Input: part model. Units: mm. Frame: model coordinates. A direction names the side the tool comes from. Coordinates: 2 decimals unless noted, no trailing zeros. Order: outer loops, then holes, each group sorted by start corner. A loop starts at its lowest first (then second) coordinate and runs counter-clockwise, first axis right, second up. Notation, with made-up numbers: M 67.5,79 L 105.5,79 A30 cw 105.5,118 Z; hole C 19.25,-14.5 d2. An arc over 180 degrees is marked long. Answer in a Markdown table with one row per item.
Autodesk Inventor part; units mm, degrees
ref_plane "YZ Plane" through (0, 0, 0) normal (1, 0, 0) x (0, 1, 0)
ref_plane "XZ Plane" through (0, 0, 0) normal (0, 1, 0) x (-1, 0, 0)
ref_plane "XY Plane" through (0, 0, 0) normal (0, 0, 1) x (1, 0, 0)
sketch "Skizze1" plane through (0, 0, 0) normal (0, 0, 1) x (1, 0, 0)
  line L0 (-8.75, -35.5) -> (8.75, -35.5)
  line L1 (8.75, -35.5) -> (8.75, 35.5)
  line L2 (8.75, 35.5) -> (-8.75, 35.5)
  line L3 (-8.75, 35.5) -> (-8.75, -35.5)
  line L4 (-8.75, -35.5) -> (8.75, 35.5) construction
  line L5 (8.75, -35.5) -> (-8.75, 35.5) construction
  point P0 (0, 0)
  dimension "d0" = 17.5
  dimension "d1" = 71
extrude "Extrusion1" add sketch "Skizze1" along normal blind 2
sketch "Skizze2" plane through (0, 0, 2) normal (0, 0, 1) x (1, 0, 0)
  circle A0 centre (-6.25, 33) radius 1.5
  line L0 (8.75, 35.5) -> (-8.75, 35.5)
  line L1 (0, 35.5) -> (0, 32.4568) construction
  circle A1 centre (6.25, 33) radius 1.5
  line L2 (-3.3034, 0) -> (2.2681, 0) construction
  circle A2 centre (-6.25, -33) radius 1.5
  circle A3 centre (6.25, -33) radius 1.5
  line L3 (-8.75, 35.5) -> (-8.75, -35.5) construction
  point P0 (0, 0)
  dimension "d4" = 3
  dimension "d5" = 2.5
  dimension "d6" = 2.5
extrude "Extrusion2" cut sketch "Skizze2" against normal blind 2
sketch "Skizze3" plane through (0, 0, 0) normal (0, 0, -1) x (-1, 0, 0)
  line L0 (8.75, 35.5) -> (8.75, -35.5)
  line L1 (-8.75, -25.5) -> (8.75, -25.5)
  line L2 (8.75, -25.5) -> (8.75, 15.5)
  line L3 (8.75, 15.5) -> (-8.75, 15.5)
  line L4 (-8.75, 15.5) -> (-8.75, -25.5)
  line L5 (-8.75, -25.5) -> (8.75, 15.5) construction
  line L6 (8.75, -25.5) -> (-8.75, 15.5) construction
  line L7 (8.75, -35.5) -> (-8.75, -35.5)
  line L8 (-8.75, -35.5) -> (-8.75, 35.5)
  point P0 (0, -5)
  point P1 (8.75, -25.5)
  dimension "d9" = 41
  dimension "d17" = 10
extrude "Extrusion3" add sketch "Skizze3" along normal blind 13 contours L0 L1 L4 L3
sketch "Skizze4" plane through (-8.75, -35.5, 2) normal (-1, 0, 0) x (0, 0, 1)
  line L0 (-2, 10) -> (-15, 10)
  line L1 (-12.32, 10) -> (-2, 10)
  line L2 (-2, 10) -> (-2, 11.25)
  line L3 (-2, 11.25) -> (-12.32, 11.25)
  line L4 (-12.32, 11.25) -> (-12.32, 10)
  line L5 (-15, 10) -> (-15, 51)
  line L6 (-4.404, 30.5) -> (2.981, 30.5) construction
  line L7 (-2, 51) -> (-15, 51)
  line L8 (-2, 51) -> (-2, 49.75)
  line L9 (-2, 49.75) -> (-12.32, 49.75)
  line L10 (-12.32, 49.75) -> (-12.32, 51)
  line L11 (-2, 10) -> (-12.32, 10)
  point P0 (-2, 35.5)
  point P1 (-12.32, 10.625)
  dimension "d12" = 2.68
  dimension "d13" = 1.25
extrude "Extrusion4" cut sketch "Skizze4" against normal blind 17.5
fillet "Rundung1" radius 1 6 edges at (-8.75, -35.5, 1) (8.75, -35.5, 1) (8.75, 35.5, 1) (-8.75, 35.5, 1) (0, 15.5, -13) (0, -25.5, -13)
properties part number "Relais_Platte_3D-Druck"
1) Mould query, pull axis Z, two halves, no side actions, for faces 1 (the face through (0, 0, 2)), 2 (the face through (0, -5, -13)), 3 (the face through (0, -25, -10.32)), 4 (the face through (5.925, 31.536, 1.014)). Classes: +Z half, -Z half, draft (parallel to the pull), parting line (faces both ways), or undercut.
Resolved:
| item | result |
|---|---|
| face 1 | +Z half |
| face 2 | -Z half |
| face 3 | undercut |
| face 4 | draft |
2) Cut plane C-C, the plane x = -2. Output: boundary loops of the cut face in (y, z).
Resolved:
| item | result |
|---|---|
| outline | M -35.5,0 L -24.25,0 L -24.25,-10.32 L -25.5,-10.32 L -25.5,-12 A1 ccw -24.5,-13 L 14.5,-13 A1 ccw 15.5,-12 L 15.5,-10.32 L 14.25,-10.32 L 14.25,0 L 35.5,0 L 35.5,2 L -35.5,2 Z |
3) Reachability of faces 5 (the face through (0, -25.5, -11)), 6 (the face through (0, 35.5, 1)), 7 (the face through (0, -24.25, -5)), 8 (the face through (0, 14.25, -5)), 9 (the face through (0, 15.5, -11)) from +Z, -Z, +X, -X, +Y, -Y: full face, straight path, thin tool, end or side. Return the list, or none.
Resolved:
| item | result |
|---|---|
| face 5 | -Z, +X, -X, -Y |
| face 6 | +Z, -Z, +X, -X, +Y |
| face 7 | +X, -X, -Y |
| face 8 | +X, -X, +Y |
| face 9 | -Z, +X, -X, +Y |
4) Cut plane A-A, the plane x = -6.25. Output: boundary loops of the cut face in (y, z), and give its area (3 significant figures).
Resolved:
| item | result |
|---|---|
| outline | M -35.5,0 L -34.5,0 L -34.5,2 L -35.5,2 Z; M -31.5,0 L -24.25,0 L -24.25,-10.32 L -25.5,-10.32 L -25.5,-12 A1 ccw -24.5,-13 L 14.5,-13 A1 ccw 15.5,-12 L 15.5,-10.32 L 14.25,-10.32 L 14.25,0 L 31.5,0 L 31.5,2 L -31.5,2 Z; M 34.5,0 L 35.5,0 L 35.5,2 L 34.5,2 Z |
| area | 637 mm2 |
5) Contact query for flat-ended pins moving along their axis: pin 1 (5 mm diameter, centred on x = -5, z = -10, fed in from -Y); pin 2 (1 mm diameter, centred on x = -5.5, z = -11.5, fed in from +Y); pin 3 (9 mm diameter, centred on x = 1, y = 21, fed in from -Z). Output: stop coordinate, or through.
Resolved:
| item | result |
|---|---|
| pin 1 | stops at y = -25.5 |
| pin 2 | stops at y = 15.5 |
| pin 3 | stops at z = 0 |
6) Cut plane B-B, the plane y = 33. Output: boundary loops of the cut face in (x, z), and give its area (3 significant figures).
Resolved:
| item | result |
|---|---|
| outline | M -8.75,0 L -7.75,0 L -7.75,2 L -8.75,2 Z; M -4.75,0 L 4.75,0 L 4.75,2 L -4.75,2 Z; M 7.75,0 L 8.75,0 L 8.75,2 L 7.75,2 Z |
| area | 23.0 mm2 |
7) Cut plane D-D, the plane z = -6.75. Output: boundary loops of the cut face in (x, y).
Resolved:
| item | result |
|---|---|
| outline | M -8.75,-24.25 L 8.75,-24.25 L 8.75,14.25 L -8.75,14.25 Z |
8) Material intervals for probe 1 along Y at (x, z) = (-6.25, 1.3); probe 2 along Z at (x, y) = (-4, 14.5); probe 3 along Z at (x, y) = (-3.25, 24.5), sorted ascending.
Resolved:
| item | result |
|---|---|
| probe 1 | y = -35.5 to -34.5, -31.5 to 31.5, 34.5 to 35.5 |
| probe 2 | z = -13 to -10.32, 0 to 2 |
| probe 3 | z = 0 to 2 |
